Autodesk Inventor part; units mm, degrees
ref_plane "YZ Plane" through (0, 0, 0) normal (1, 0, 0) x (0, 1, 0)
ref_plane "XZ Plane" through (0, 0, 0) normal (0, 1, 0) x (-1, 0, 0)
ref_plane "XY Plane" through (0, 0, 0) normal (0, 0, 1) x (1, 0, 0)
sketch "Skizze1" plane through (0, 0, 0) normal (0, 0, 1) x (1, 0, 0)
  circle A0 centre (-16.6663, 54.3) radius 1.65
  circle A1 centre (-5.6501, 4) radius 1.4
  circle A2 centre (-5.6501, -4) radius 1.4
  circle A3 centre (-16.9417, 18.1) radius 1.65
  line L0 (-0.6501, -22.5) -> (-10.6501, -22.5)
  line L1 (-10.6501, -22.5) -> (-10.6501, 22.5)
  line L2 (-10.6501, 22.5) -> (-0.6501, 22.5)
  line L3 (-0.6501, 22.5) -> (-0.6501, -22.5)
  line L4 (-0.6501, -22.5) -> (-10.6501, 22.5) construction
  line L5 (-10.6501, -22.5) -> (-0.6501, 22.5) construction
  point P0 (0, 0)
  point P1 (-5.6501, 0)
  dimension "d0" = 10
  dimension "d1" = 45
extrude "Extrusion1" add sketch "Skizze1" along normal blind 5 contours L0 L1 L2 L3
sketch "Skizze2" plane through (-10.6501, -22.5, 0) normal (0, -1, 0) x (1, 0, 0)
  line L0 (0, 0) -> (10, 0)
  line L1 (10, 0) -> (10, 5)
  line L2 (0, 5) -> (10, 5)
  line L3 (0, 0) -> (0, 5)
  line L4 (0, 0) -> (-1.6429, 0) construction
  line L5 (-1.6429, 0) -> (-2.7402, 4.5123) construction
  line L6 (-2.7402, 4.5123) -> (-5.3021, 5.5945) construction
  line L7 (-5.3021, 5.5945) -> (-9.43, 7.7902) construction
  line L8 (-9.43, 7.7902) -> (-13.8799, 3.8379) construction
  line L9 (-13.8799, 3.8379) -> (-13.7228, -1.3116) construction
  spline S0 degree 4 poles (0, 0) (-1.6429, 0) (-2.7402, 4.5123) (-5.3021, 5.5945) (-9.43, 7.7902) (-13.8799, 3.8379) (-13.7228, -1.3116) knots 1 1 1 1 1 2 3 4 4 4 4 4
  line L10 (0, 5) -> (-0.4655, 5) construction
  line L11 (-0.4655, 5) -> (-2.7402, 8.0244) construction
  line L12 (-2.7402, 8.0244) -> (-7.1757, 9.8395) construction
  line L13 (-7.1757, 9.8395) -> (-10.7181, 10.2483) construction
  line L14 (-10.7181, 10.2483) -> (-17.7424, 4.5123) construction
  line L15 (-17.7424, 4.5123) -> (-17.7424, -1.3116) construction
  spline S1 degree 4 poles (0, 5) (-0.4655, 5) (-2.7402, 8.0244) (-7.1757, 9.8395) (-10.7181, 10.2483) (-17.7424, 4.5123) (-17.7424, -1.3116) knots 1 1 1 1 1 2 3 4 4 4 4 4
  line L16 (-17.7424, -1.3116) -> (-13.7228, -1.3116)
  point P0 (10.6501, 0)
extrude "Extrusion2" add sketch "Skizze2" against normal up to surface (45 mm away) contours S0 L16 S1 L3
sketch "Skizze3" plane through (0, 0, 5) normal (0, 0, 1) x (1, 0, 0)
  line L0 (-0.6501, 22.5) -> (-10.6501, 22.5)
  line L1 (-10.6501, 22.5) -> (-10.6501, -22.5)
  line L2 (-10.6501, -22.5) -> (-0.6501, -22.5)
  line L3 (-0.6501, -22.5) -> (-0.6501, 22.5)
  circle A0 centre (-5.6501, -4) radius 1.4
  circle A1 centre (-5.6501, 4) radius 1.4
  line L4 (-42.8998, -7.5) -> (-10.6501, -7.5)
  line L5 (-10.6501, -7.5) -> (-10.6501, 7.5)
  line L6 (-10.6501, 7.5) -> (-42.8998, 7.5)
  line L7 (-42.8998, 7.5) -> (-42.8998, -7.5)
  line L8 (-42.8998, -7.5) -> (-10.6501, 7.5) construction
  line L9 (-10.6501, -7.5) -> (-42.8998, 7.5) construction
  line L10 (-10.6501, 22.5) -> (-42.8998, 7.5)
  line L11 (-42.8998, -7.5) -> (-10.6501, -22.5)
  line L12 (-42.8998, 22.5) -> (-10.6501, 22.5)
  line L13 (-10.6501, 22.5) -> (-10.6501, -22.5)
  line L14 (-10.6501, -22.5) -> (-42.8998, -22.5)
  line L15 (-42.8998, -22.5) -> (-42.8998, 22.5)
  point P0 (0, 0)
  point P1 (-26.775, 0)
  point P2 (-10.6501, -7.5)
  dimension "d6" = 15
extrude "Extrusion3" cut sketch "Skizze3" along normal through all both and the other way through all contours L1 L4 L7 L6
fillet "Rundung1" radius 2 2 edges at (-10.6501, 7.5, 2.5) (-10.6501, -7.5, 2.5)
properties part number "60_Planktoscope_Sampleclamp"
For this review, take the finished solid that the model builds, in its own axes (mm). A direction names the side the tool comes from. Coordinates: 2 decimals unless noted, no trailing zeros. Loops run counter-clockwise (first coordinate to the right, second up) from the corner with the lowest first, then second, coordinate; pieces in that order, holes last. Notation, with made-up numbers: (49, 11) - (88, 11) arc R19 ccw to (88, 17) - close; hole circle Ø6 at (0.5, -35). An arc over 180 degrees is marked (long way). Use a Markdown table: item, result. Add a question column.
Item 1: Mouldability with a two-part tool opening along X and no side actions: class faces 1 (the face through (-5.954, -2.633, 2.465)), 2 (the face through (-11.22, -6.9, 2.55)), 3 (the face through (-15, 22.5, 6)) as pulls with the +X half, pulls with the -X half, needs draft (parallel to the pull), parting line crosses it, or undercut.
Item 2: For line 1 (Y direction, x = -5, z = 2); line 2 (Y direction, x = -19.5, z = 7.75); line 3 (X direction, y = -2.5, z = 1.5), list the stretches that pass through material, from the lowest coordinate up.
Item 3: Tool access review of faces 4 (the face through (-22.4, -7.5, 5.3)), 5 (the face through (-6, 0, 0)), 6 (the face through (-6, 0, 5)), 7 (the face through (-14, -22.5, 6)): name each direction out of +Z, -Z, +X, -X, +Y, -Y from which nothing blocks a thin tool from reaching the whole face with its end or side.
Item 4: We need section A-A (y = 4). Give the boundary of the cut face in (x, z), and give its area (3 significant figures).
Item 5: Insertion check: pin 1 Ø1.5 at (y, z) = (14.5, 8) entering from +X; pin 2 Ø5 at (x, y) = (-12.5, 2) entering from +Z; pin 3 Ø3 at (y, z) = (0.5, 3.5) entering from -X; pin 4 Ø5.5 at (x, z) = (-19, 2.5) entering from -Y. Each pin has a flat end and moves straight along its axis. Give the tip position at first contact, or say it passes through.
Item 6: We need section B-B (x = -6.25). Give the boundary of the cut face in (y, z), and give its area (3 significant figures).
Results list:
| question | item | result |
|---|---|---|
| 1 | face 1 | undercut |
| 1 | face 2 | pulls with the -X half |
| 1 | face 3 | needs draft |
| 2 | line 1 | y = -22.5 to -5.24, -2.76 to 2.76, 5.24 to 22.5 |
| 2 | line 2 | y = -22.5 to -7.5, 7.5 to 22.5 |
| 2 | line 3 | x = -10.65 to -0.65 |
| 3 | face 4 | +Z, -Z, -X |
| 3 | face 5 | -Z, +X, +Y, -Y |
| 3 | face 6 | +Z, +X, +Y, -Y |
| 3 | face 7 | +Z, -Z, +X, -X, -Y |
| 4 | outline | (-10.65, 0) - (-7.05, 0) - (-7.05, 5) - (-10.65, 5) - close; (-4.25, 0) - (-0.65, 0) - (-0.65, 5) - (-4.25, 5) - close |
| 4 | area | 36.0 mm^2 |
| 5 | pin 1 | stops at x = -13.32 |
| 5 | pin 2 | stops at z = 5 |
| 5 | pin 3 | stops at x = -10.65 |
| 5 | pin 4 | passes through |
| 6 | outline | (-22.5, 0) - (-5.26, 0) - (-5.26, 5) - (-22.5, 5) - close; (-2.74, 0) - (2.74, 0) - (2.74, 5) - (-2.74, 5) - close; (5.26, 0) - (22.5, 0) - (22.5, 5) - (5.26, 5) - close |
| 6 | area | 200 mm^2 |
